from build123d import *

# Parameters (mm, degrees)
SKETCH1_R           = 26
SKETCH1_R_2         = 4.2
SKETCH1_R_3         = 1.275
BOSS_EXTRUDE1_DEPTH = 2.5
SKETCH2_R           = 5.1
CUT_EXTRUDE1_DEPTH  = 1.4
FILLET1_R           = 0.2
FILLET2_R           = 1


with BuildPart() as part:
    # Sketch1 → Boss-Extrude1 (new body)
    with BuildSketch(Plane.XY):
        Circle(SKETCH1_R)
        Circle(SKETCH1_R_2, mode=Mode.SUBTRACT)
        with Locations((0, -7.75)):
            Circle(SKETCH1_R_3, mode=Mode.SUBTRACT)
        with Locations((-6.711696879, 3.875)):
            Circle(SKETCH1_R_3, mode=Mode.SUBTRACT)
        with Locations((6.711696879, 3.875)):
            Circle(SKETCH1_R_3, mode=Mode.SUBTRACT)
    extrude(amount=BOSS_EXTRUDE1_DEPTH)

    # Sketch2 → Cut-Extrude1 (cut)
    with BuildSketch(Plane.XY.offset(2.5)):
        Circle(SKETCH2_R)
    extrude(amount=-CUT_EXTRUDE1_DEPTH, mode=Mode.SUBTRACT)

    # Fillet1
    fillet1_edges = [part.edges().sort_by_distance(p)[0] for p in [
        (-5.1, 0, 2.5),
    ]]
    fillet(fillet1_edges, radius=FILLET1_R)

    # Fillet2
    fillet2_edges = [part.edges().sort_by_distance(p)[0] for p in [
        (-26, 0, 0),
    ]]
    fillet(fillet2_edges, radius=FILLET2_R)


solid = part.part
Can you work these out from the model? Positions are in its coordinate system, mm. A direction names the side the tool comes from. Give positions to 0.01 mm unless a question says otherwise; leave off trailing zeros. Loops run counter-clockwise (first coordinate to the right, second up) from the corner with the lowest first, then second, coordinate; pieces in that order, holes last. Notation, with made-up numbers: (-24.75, 79.5) -> (-18.75, 79.5) arc R16 cw to (-18.75, 90.5) -> close; hole circle Ø8 at (-17.5, -3.75). An arc over 180 degrees is marked (long way). Use one line per item in the form item = value.
1) If we section it at B-B (y = 0): Please give me the cut outline in (x, z), plus the area to 3 significant figures.
Answers:
outline = (-26, 1) arc R1 ccw to (-25, 0) -> (-4.2, 0) -> (-4.2, 1.1) -> (-5.1, 1.1) -> (-5.1, 2.3) arc R0.2 ccw to (-5.3, 2.5) -> (-26, 2.5) -> close; (4.2, 0) -> (25, 0) arc R1 ccw to (26, 1) -> (26, 2.5) -> (5.3, 2.5) arc R0.2 ccw to (5.1, 2.3) -> (5.1, 1.1) -> (4.2, 1.1) -> close
area = 106 mm²
2) For faces 1 (the face through (7.3, 2.744, 1.232)), 2 (the face through (-2, 4, 1.1)), which set-ups out of +Z, -Z, +X, -X, +Y, -Y let a thin tool reach every point of the face, with its end or its side?
Answers:
face_1 = +Z, -Z
face_2 = +Z
3) We'd pull the mould along Y, two halves only. Please class faces 3 (the face through (0, -5, 0)), 4 (the face through (2.4, -4.5, 1.7)), 5 (the face through (-20.633, -15.821, 1.74)): released by +Y, released by -Y, zero draft, split by the parting line, or undercut.
Answers:
face_3 = zero draft
face_4 = undercut
face_5 = split by the parting line
4) I need wall thicknesses on line 1 along Y through (x, z) = (0, 1.7) (3 decimals); line 2 along Y through (x, z) = (0, 0.2) (3 decimals); line 3 along Y through (x, z) = (-6, 1.35). Which ranges of each line are inside material? Lowest first, please.
Answers:
line_1 = -26 to -9.025, -6.475 to -5.1, 5.1 to 26
line_2 = -25.6 to -9.025, -6.475 to -4.2, 4.2 to 25.6
line_3 = -25.3 to 2.82, 4.93 to 25.3
5) If we section it at A-A (x = 0): Please give me the cut outline in (y, z) (3 decimals), plus the area to 3 significant figures.
Answers:
outline = (-26, 1) arc R1 ccw to (-25, 0) -> (-9.025, 0) -> (-9.025, 2.5) -> (-26, 2.5) -> close; (-6.475, 0) -> (-4.2, 0) -> (-4.2, 1.1) -> (-5.1, 1.1) -> (-5.1, 2.3) arc R0.2 ccw to (-5.3, 2.5) -> (-6.475, 2.5) -> close; (4.2, 0) -> (25, 0) arc R1 ccw to (26, 1) -> (26, 2.5) -> (5.3, 2.5) arc R0.2 ccw to (5.1, 2.3) -> (5.1, 1.1) -> (4.2, 1.1) -> close
area = 99.7 mm²
6) Will this pin go through, and if not, where does the flat tip stop? pin 1 (1 mm diameter, centred on x = 15.5, z = 1.5, fed in from -Y).
Answers:
pin_1 = -21.24
